Work out the finished part from the listing and answer in its coordinate system (mm). Round coordinates to 2 decimals unless told otherwise and drop trailing zeros. Order: outer loops, then holes, each group sorted by start corner. A loop starts at its lowest first (then second) coordinate and runs counter-clockwise, first axis right, second up. Notation, with made-up numbers: (-23, 37.25) - (31, 37.25) arc R19 cw to (31, 48.25) - close; hole circle Ø9 at (-8.5, 66). An arc over 180 degrees is marked (long way). Use one line per item in the form item = value. Start each with the question number.
Q1. The part is cut by section B-B on y = 130.5. Determine the outline of the cut face in (x, z) (3 decimals).
Q2. The part is cut by section C-C on z = 44. Determine the outline of the cut face in (x, y) (3 decimals), plus the area to 3 significant figures.
Q3. Find the intervals of material crossed by line 1 (Z direction, x = 0.3, y = 93.5); line 2 (Y direction, x = 0.6, z = 186); line 3 (Z direction, x = 1.8, y = 102.5), in increasing order. Write a range as [from, to].
Q4. Given P1, Ø1.6, axis at x = 1.5, z = 30, coming from the -Y side; P2, Ø1.6, axis at x = 2, y = 136, coming from the -Z side; P3, Ø0.7, axis at x = 2, z = 205.5, coming from the -Y side, each flat-ended and moving along its own axis, determine where each tip first touches the part or whether it passes through.
Q5. The part is cut by section A-A on x = 0.7. Determine the outline of the cut face in (y, z), plus the area to 3 significant figures.
from build123d import *

# Parameters (mm, degrees)
BOSS_EXTRUDE1_DEPTH     = 3.175
CUT_EXTRUDE1_DEPTH      = 273.554100881
CUT_EXTRUDE1_DEPTH_BACK = 273.554100881


with BuildPart() as part:
    # Sketch1 → Boss-Extrude1 (new body)
    with BuildSketch(Plane(origin=(0, 0, 0), x_dir=(0, 0, -1), z_dir=(1, 0, 0))):
        with BuildLine():
            Line((-202.720111625, -68.875155483), (-185.257611625, -68.875155483))
            Line((-185.257611625, -68.875155483), (-185.257611625, -72.050155483))
            Line((-185.257611625, -72.050155483), (-124.932611625, -72.050155483))
            Line((-124.932611625, -72.050155483), (-124.932611625, -68.875155483))
            Line((-124.932611625, -68.875155483), (124.932611625, -68.875155483))
            Line((124.932611625, -68.875155483), (139.862388375, -68.875155483))
            Line((139.862388375, -68.875155483), (139.862388375, -72.050155483))
            Line((139.862388375, -72.050155483), (200.187388375, -72.050155483))
            Line((200.187388375, -72.050155483), (200.187388375, -68.875155483))
            Line((200.187388375, -68.875155483), (220.824888375, -68.875155483))
            Line((220.824888375, -68.875155483), (220.824888375, 69.554844517))
            Line((220.824888375, 69.554844517), (220.189888375, 69.554844517))
            ThreePointArc((220.189888375, 69.554844517), (218.393837151, 70.298793293), (217.649888375, 72.094844517))
            Line((217.649888375, 72.094844517), (217.649888375, 159.724844517))
            Line((217.649888375, 159.724844517), (17.624888375, 159.724844517))
            Line((17.624888375, 159.724844517), (17.624888375, 94.954844517))
            Line((17.624888375, 94.954844517), (-202.720111625, 94.954844517))
            Line((-202.720111625, 94.954844517), (-202.720111625, 70.824844517))
            ThreePointArc((-202.720111625, 70.824844517), (-203.4640604, 69.028793293), (-205.260111625, 68.284844517))
            Line((-205.260111625, 68.284844517), (-205.895111625, 68.284844517))
            Line((-205.895111625, 68.284844517), (-205.895111625, -59.985155483))
            Line((-205.895111625, -59.985155483), (-205.260111625, -59.985155483))
            ThreePointArc((-205.260111625, -59.985155483), (-203.4640604, -60.729104259), (-202.720111625, -62.525155483))
            Line((-202.720111625, -62.525155483), (-202.720111625, -68.875155483))
        make_face()
    extrude(amount=BOSS_EXTRUDE1_DEPTH)

    # Sketch2 → Cut-Extrude1 (cut, two sides: drawn at the far end of the back side and taken through both)
    with BuildSketch(Plane(origin=(3.175, 0, 0), x_dir=(0, 0, -1), z_dir=(1, 0, 0)).offset(-CUT_EXTRUDE1_DEPTH_BACK)):
        with BuildLine():
            Line((220.824888375, -68.875155483), (217.649888375, -68.875155483))
            Line((217.649888375, -68.875155483), (217.649888375, -62.525155483))
            ThreePointArc((217.649888375, -62.525155483), (218.393837151, -60.729104259), (220.189888375, -59.985155483))
            Line((220.189888375, -59.985155483), (220.824888375, -59.985155483))
            Line((220.824888375, -59.985155483), (220.824888375, -68.875155483))
        make_face()
    extrude(amount=CUT_EXTRUDE1_DEPTH + CUT_EXTRUDE1_DEPTH_BACK, mode=Mode.SUBTRACT)


solid = part.part
Found:
q1.outline = (0, -217.65) - (3.175, -217.65) - (3.175, -17.625) - (0, -17.625) - close
q2.outline = (0, -68.875) - (3.175, -68.875) - (3.175, 94.955) - (0, 94.955) - close
q2.area = 520 mm²
q3.line_1 = [-217.65, 202.72]
q3.line_2 = [-68.88, 94.95]
q3.line_3 = [-217.65, -17.62]
q4.P1 = -68.88
q4.P2 = -217.65
q4.P3 = -59.99
q5.outline = (-72.05, -200.19) - (-68.88, -200.19) - (-68.88, -217.65) - (-62.53, -217.65) arc R2.54 cw to (-59.99, -220.19) - (-59.99, -220.82) - (69.55, -220.82) - (69.55, -220.19) arc R2.54 cw to (72.09, -217.65) - (159.72, -217.65) - (159.72, -17.62) - (94.95, -17.62) - (94.95, 202.72) - (70.82, 202.72) arc R2.54 cw to (68.28, 205.26) - (68.28, 205.9) - (-59.99, 205.9) - (-59.99, 205.26) arc R2.54 cw to (-62.53, 202.72) - (-68.88, 202.72) - (-68.88, 185.26) - (-72.05, 185.26) - (-72.05, 124.93) - (-68.88, 124.93) - (-68.88, -139.86) - (-72.05, -139.86) - close
q5.area = 83,000 mm²
